For this review, use the dimensioned drawing (mm, ordinates from the lowest corner) and the shaded views. A direction names the side the tool comes from. Round coordinates to 2 decimals unless told otherwise and drop trailing zeros. Order: outer loops, then holes, each group sorted by start corner. A loop starts at its lowest first (then second) coordinate and runs counter-clockwise, first axis right, second up. Notation, with made-up numbers: M 71.25,-21.75 L 122.25,-21.75 A6 cw 122.25,-14.75 Z; hole C 42,41 d9. An arc over 180 degrees is marked long. Use a Markdown table: item, result. Add a question column.
1. For the marked faces 1 and 2, list the 3-axis set-ups (+Z, -Z, +X, -X, +Y, -Y) from which the entire face can be reached by the end or side of a thin tool; tool diameter is ignored.
2. Insertion check: P1, Ø10, axis at x = 50.5, y = 34, coming from the +Z side (3 decimals); P2, Ø2, axis at x = 38, z = 22.5, coming from the +Y side; P3, Ø5, axis at x = 34, y = 34, coming from the -Z side. Each pin has a flat end and moves straight along its axis. Give the tip position at first contact, or say it passes through.
3. To check wall thickness, follow probe 1 along X at (y, z) = (3.5, 11); probe 2 along Y at (x, z) = (28.5, 46); probe 3 along Z at (x, y) = (69.5, 56) (1 decimal). State the ranges of each line that lie inside material, in increasing order.
4. Consider section C-C on x = 31. State the section outline as (y, z) points (1 decimal).
5. Consider section A-A on z = 31. State the section outline as (x, y) points.
6. Consider section B-B on y = 50.5. State the section outline as (x, z) points (1 decimal), then the cut area to 3 significant figures.
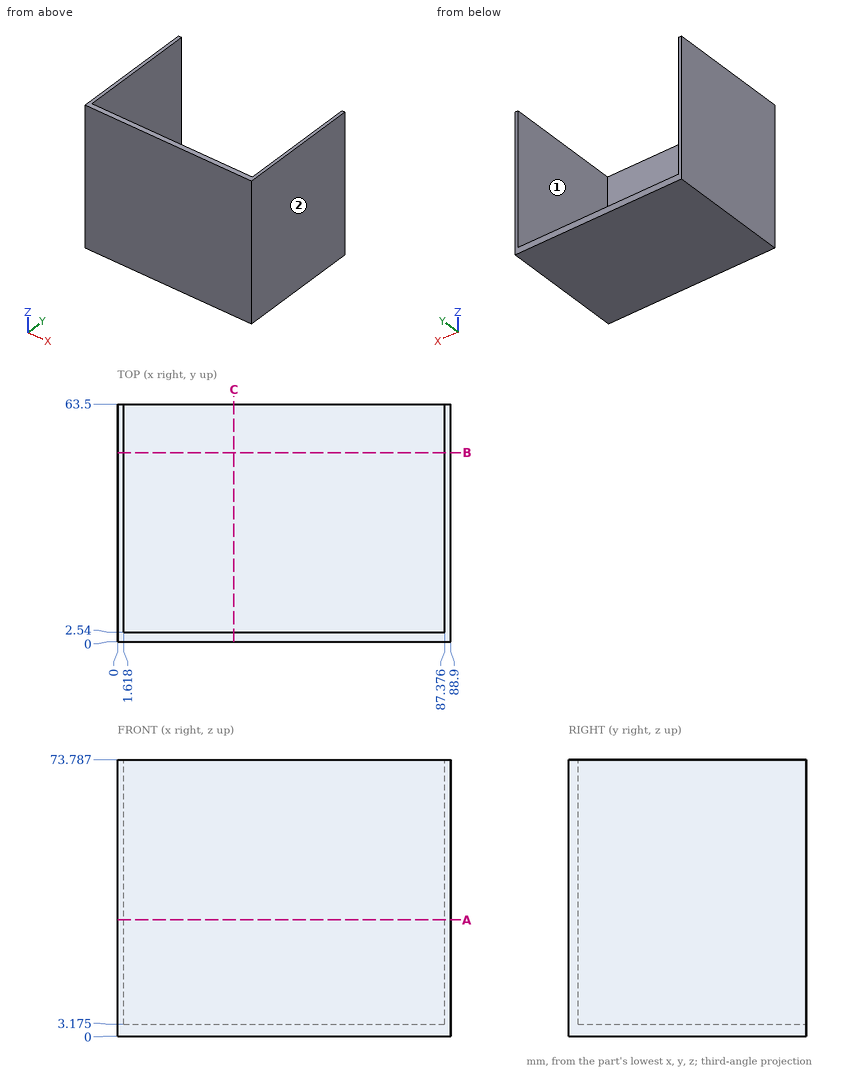
Answer block:
| question | item | result |
|---|---|---|
| 1 | face 1 | +Z, +Y |
| 1 | face 2 | +Z, -Z, +X, +Y, -Y |
| 2 | P1 | z = 3.175 |
| 2 | P2 | y = 2.54 |
| 2 | P3 | z = 0 |
| 3 | probe 1 | 0 to 1.62, 87.38 to 88.9 |
| 3 | probe 2 | 0 to 2.54 |
| 3 | probe 3 | 0 to 3.2 |
| 4 | outline | M 0,0 L 63.5,0 L 63.5,3.2 L 2.5,3.2 L 2.5,73.8 L 0,73.8 Z |
| 5 | outline | M 0,0 L 88.9,0 L 88.9,63.5 L 87.38,63.5 L 87.38,2.54 L 1.62,2.54 L 1.62,63.5 L 0,63.5 Z |
| 6 | outline | M 0,0 L 88.9,0 L 88.9,73.8 L 87.4,73.8 L 87.4,3.2 L 1.6,3.2 L 1.6,73.8 L 0,73.8 Z |
| 6 | area | 504 mm^2 |
